Source: CAD feature listing. Evaluate the final solid. Frame: model axes, mm. Face numbers are marked on the shaded views. A direction names the side the tool comes from. Coordinates: 2 decimals unless noted, no trailing zeros. Loops run counter-clockwise (first coordinate to the right, second up) from the corner with the lowest first, then second, coordinate; pieces in that order, holes last.
from build123d import *

# Parameters (mm, degrees)
SM_BASE_FLANGE_1_DEPTH   = 15.5
OTHER_START              = -23.68807717
OTHER_1_OUTLINE_W        = 1.5
OTHER_1_OUTLINE_H        = 10
OTHER_1_DEPTH            = 3.535533906
SKETCH_6_R               = 5.5
CUT_EXTRUDE_752_DEPTH    = 68.329414077
SKETCH_8_W               = 57
SKETCH_8_H               = 17
SM_BASE_FLANGE_1_2_DEPTH = 1.5
SKETCH_7_R               = 3.5
CUT_EXTRUDE_2_DEPTH      = 10
SKETCH_9_W               = 11
SKETCH_9_H               = 9
SM_BASE_FLANGE_2_DEPTH   = 1.5
SKETCH_12_W              = 11
SKETCH_12_H              = 9
SM_BASE_FLANGE_3_DEPTH   = 1.5


# Read off the part's stored shape, not the designer's step: Затупленный угол1
# Sheet-metal steps are written as plain solids
with BuildPart() as part:
    # Sketch 1 → Sm Base Flange 1 (new, symmetric)
    with BuildSketch(Plane.XY):
        with BuildLine():
            Line((-30, -18), (-30, -1.5))
            ThreePointArc((-30, -1.5), (-29.560660172, -0.439339828), (-28.5, 0))
            Line((-28.5, 0), (28.5, 0))
            ThreePointArc((28.5, 0), (29.560660172, -0.439339828), (30, -1.5))
            Line((30, -1.5), (30, -18))
            Line((30, -18), (31.5, -18))
            Line((31.5, -18), (31.5, -1.5))
            ThreePointArc((31.5, -1.5), (30.621320344, 0.621320344), (28.5, 1.5))
            Line((28.5, 1.5), (-28.5, 1.5))
            ThreePointArc((-28.5, 1.5), (-30.621320344, 0.621320344), (-31.5, -1.5))
            Line((-31.5, -1.5), (-31.5, -18))
            Line((-31.5, -18), (-30, -18))
        make_face()
    extrude(amount=SM_BASE_FLANGE_1_DEPTH, both=True)

    # Other 1 outline → Other 1 (cut)
    with BuildSketch(Plane(origin=(0, 0, 0), x_dir=(1, 0, 0), z_dir=(0, 0.7071067811865476, 0.7071067811865476)).offset(OTHER_START)):
        with Locations((-30.75, -2)):
            Rectangle(OTHER_1_OUTLINE_W, OTHER_1_OUTLINE_H)
        with Locations((30.75, -2)):
            Rectangle(OTHER_1_OUTLINE_W, OTHER_1_OUTLINE_H)
    extrude(amount=OTHER_1_DEPTH, mode=Mode.SUBTRACT)

    # Эскиз6 → Cut-Extrude 752 (cut, through all)
    with BuildSketch(Plane.ZY.offset(31.5)):
        with Locations((-7.5, -10)):
            Circle(SKETCH_6_R)
    extrude(amount=-CUT_EXTRUDE_752_DEPTH, mode=Mode.SUBTRACT)

    # Эскиз8 → Sm Base Flange 1 2 (add)
    with BuildSketch(Plane(origin=(0, 1.5, 0), x_dir=(1, 0, 0), z_dir=(0, 1, 0))):
        with Locations((0, -24)):
            Rectangle(SKETCH_8_W, SKETCH_8_H)
    extrude(amount=-SM_BASE_FLANGE_1_2_DEPTH)

    # Эскиз7 → Вырез-Вытянуть2 (cut)
    with BuildSketch(Plane(origin=(0, 1.5, 0), x_dir=(1, 0, 0), z_dir=(0, 1, 0))):
        with Locations(Location((-15, -22.5, 0), (0, 0, 270))):
            Circle(SKETCH_7_R)
        with Locations(Location((15, -22.5, 0), (0, 0, 90))):
            Circle(SKETCH_7_R)
    extrude(amount=-CUT_EXTRUDE_2_DEPTH, mode=Mode.SUBTRACT)

    # Эскиз9 → Выступ2 (add)
    with BuildSketch(Plane(origin=(31.5, 0, 0), x_dir=(0, 0, -1), z_dir=(1, 0, 0))):
        with Locations((-10, -22.5)):
            Rectangle(SKETCH_9_W, SKETCH_9_H)
    extrude(amount=-SM_BASE_FLANGE_2_DEPTH)

    # Эскиз12 → Выступ3 (add)
    with BuildSketch(Plane.ZY.offset(31.5)):
        with Locations((10, -22.5)):
            Rectangle(SKETCH_12_W, SKETCH_12_H)
    extrude(amount=-SM_BASE_FLANGE_3_DEPTH)


solid = part.part
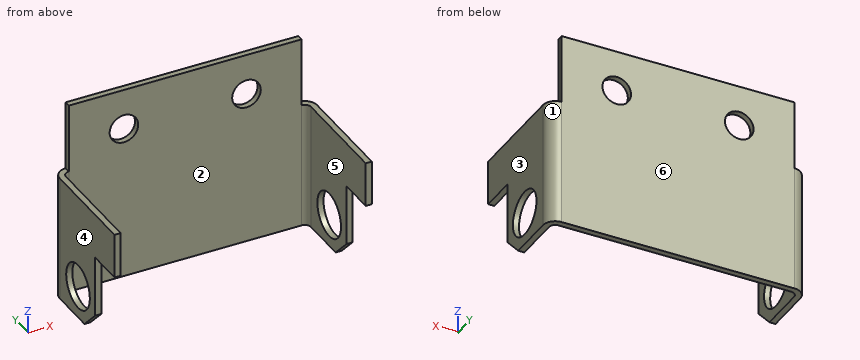
Q1. Section A-A, the plane x = 15. Return the cut outline in (y, z), plus the area to 3 significant figures.
Q2. Section C-C, the plane z = 22.5. Return the cut outline in (x, y), plus the area to 3 significant figures.
Q3. Section D-D, the plane y = -10. Return the cut outline in (x, z), plus the area to 3 significant figures.
Q4. Section B-B, the plane y = -22.25. Return the cut outline in (x, z).
Q5. Contact query for flat-ended pins moving along their axis: pin 1 Ø1.2 at (x, y) = (30.5, -20.5) entering from -Z; pin 2 Ø1.2 at (x, z) = (31, -1) entering from -Y; pin 3 Ø1.2 at (y, z) = (0.5, 27) entering from +X. Output: stop coordinate, or through.
Q6. Access query for the marked faces 1 and 2. Directions: +Z, -Z, +X, -X, +Y, -Y. A direction counts if a zero-diameter tool reaches every point of the face in a straight line with its end or side. Return the directions, or none.
Q7. Line query: line 1 along X through (y, z) = (-2.25, 4); line 2 along Y through (x, z) = (22.5, 17.5); line 3 along Y through (x, z) = (-31, -7.5). Output: solid intervals per line, ascending.
Q8. Draft query along X for the marked faces 3, 4, 5 and 6. Return one class per face: +X half, -X half, draft (parallel to the pull), parting line (faces both ways), or undercut.
Derived:
1. outline: (0, -15.5) - (1.5, -15.5) - (1.5, 19) - (0, 19) - close; (0, 26) - (1.5, 26) - (1.5, 32.5) - (0, 32.5) - close
1. area: 61.5 mm2
2. outline: (-28.5, 0) - (-18.5, 0) - (-18.5, 1.5) - (-28.5, 1.5) - close; (-11.5, 0) - (11.5, 0) - (11.5, 1.5) - (-11.5, 1.5) - close; (18.5, 0) - (28.5, 0) - (28.5, 1.5) - (18.5, 1.5) - close
2. area: 64.5 mm2
3. outline: (-31.5, -15.5) - (-30, -15.5) - (-30, -13) - (-31.5, -13) - close; (-31.5, -2) - (-30, -2) - (-30, 15.5) - (-31.5, 15.5) - close; (30, -15.5) - (31.5, -15.5) - (31.5, -13) - (30, -13) - close; (30, -2) - (31.5, -2) - (31.5, 15.5) - (30, 15.5) - close
3. area: 60.0 mm2
4. outline: (-31.5, 4.5) - (-30, 4.5) - (-30, 15.5) - (-31.5, 15.5) - close; (30, 4.5) - (31.5, 4.5) - (31.5, 15.5) - (30, 15.5) - close
5. pin 1: stops at z = 4.5
5. pin 2: stops at y = -18
5. pin 3: stops at x = 28.5
6. face 1: +Z, -Z, +X, +Y
6. face 2: +Z, -Z, -Y
7. line 1: x = -31.5 to -30, 30 to 31.5
7. line 2: y = 0 to 1.5
7. line 3: y = -18 to -15.5, -4.5 to 0.16
8. face 3: +X half
8. face 4: -X half
8. face 5: undercut
8. face 6: draft
